Autodesk Inventor part; units mm, degrees
ref_plane "YZ Plane" through (0, 0, 0) normal (1, 0, 0) x (0, 1, 0)
ref_plane "XZ Plane" through (0, 0, 0) normal (0, 1, 0) x (-1, 0, 0)
ref_plane "XY Plane" through (0, 0, 0) normal (0, 0, 1) x (1, 0, 0)
sketch "Sketch1" plane through (0, 0, 0) normal (0, 0, 1) x (1, 0, 0)
  line L0 (-12, 5) -> (12, 5)
  line L1 (12, 5) -> (12, -5)
  line L2 (12, -5) -> (-12, -5)
  line L3 (-12, -5) -> (-12, 5)
  point P0 (0, 0)
  dimension "d0" = 24
  dimension "d1" = 10
  dimension "d2" = 5
  dimension "d3" = 12
extrude "Extrusion1" add sketch "Sketch1" along normal blind 28
sketch "Sketch2" plane through (-12, 5, 0) normal (0, 1, 0) x (1, 0, 0)
  line L0 (0, 0) -> (24, 0)
  line L1 (0, 0) -> (0, -28)
  line L2 (24, -28) -> (0, -28)
  line L3 (24, 0) -> (24, -28)
  circle A0 centre (12, -14) radius 7.5
  point P0 (12, 0)
  dimension "d6" = 15
  dimension "d7" = 28
  dimension "d8" = 24
  dimension "d9" = 12
  dimension "d10" = 14
extrude "Extrusion2" cut sketch "Sketch2" against normal up to next contours A0
sketch "Sketch7" plane through (-12, 5, 28) normal (0, 1, 0) x (1, 0, 0)
  circle A0 centre (12, 14) radius 7.5
  line L0 (0, 28) -> (0, 0)
  line L1 (24, 0) -> (0, 0)
  line L2 (24, 28) -> (24, 0)
  arc A1 (0, 14) -> (24, 14) centre (12, 14) ccw
  line L3 (24, 32) -> (24, 0)
  line L4 (24, 32) -> (24, 0)
  line L5 (24, 14) -> (24, 0)
  line L6 (24, 0) -> (0, 0)
  line L7 (24, 0) -> (0, 0)
  line L8 (0, 0) -> (0, 14)
  line L9 (0, 32) -> (0, 0)
  line L10 (0, 28) -> (24, 28)
  point P0 (12, 28)
extrude "Extrusion6" cut sketch "Sketch7" against normal blind 20 contours A1 L2 L1 L0
sketch "Sketch9" plane through (-12, -5, 0) normal (-1, 0, 0) x (0, 0, 1)
  line L0 (14, 0) -> (14, 10) construction
  line L1 (0, 10) -> (14, 10) construction
  line L2 (0, 0) -> (0, 10) construction
  line L3 (0, 0) -> (14, 0) construction
  line L4 (0, 10) -> (14, 10)
  line L5 (0, 10) -> (0, 20)
  line L6 (0, 20) -> (4, 20)
  line L7 (4, 20) -> (4, 30)
  line L8 (4, 30) -> (6, 30)
  line L9 (6, 30) -> (6, 18)
  line L10 (6, 18) -> (2, 18)
  line L11 (2, 18) -> (2, 10)
  line L12 (0, 10) -> (2, 10)
  point P0 (0, 5)
  dimension "d32" = 10
  dimension "d33" = 4
  dimension "d34" = 10
  dimension "d35" = 2
  dimension "d36" = 2
  dimension "d37" = 2
extrude "Extrusion8" add sketch "Sketch9" against normal up to surface (24 mm away)
equation "\"d9\" = 0.5 * d8"
equation "\"d10\" = 0.5 * d7"
properties part number "ProbeMount"
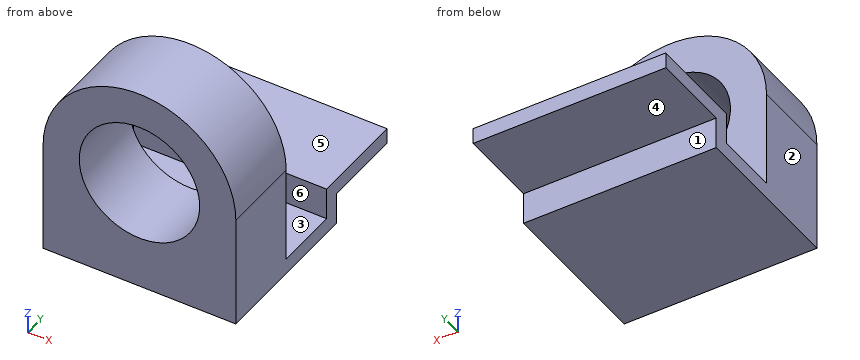
Work out the finished part from the listing and answer in its coordinate system (mm). Face numbers are marked on the shaded views. A direction names the side the tool comes from. Give positions to 0.01 mm unless a question says otherwise; leave off trailing zeros. Order: outer loops, then holes, each group sorted by start corner. A loop starts at its lowest first (then second) coordinate and runs counter-clockwise, first axis right, second up. Notation, with made-up numbers: (-18.5, 82) -> (27.5, 82) arc R24 ccw to (27.5, 118) -> close; hole circle Ø8 at (11, 87.5). An arc over 180 degrees is marked (long way). Answer as a JSON object with one key per item and string values. Group by question number.
1. A tool of negligible diameter and unlimited length cuts with its end or side. For the marked faces 4, 5 and 6, from which of +Z, -Z, +X, -X, +Y, -Y can it reach the whole face along a straight path? Write none if from no direction.
2. Flat-ended cylindrical pins translate along their axes: pin 1 Ø4 at (x, y) = (-8.5, 10.5) entering from +Z; pin 2 Ø1.2 at (x, z) = (-4, 2) entering from +Y; pin 3 Ø1.5 at (x, z) = (2, 20) entering from +Y; pin 4 Ø9.5 at (x, y) = (-3.5, 21.5) entering from +Z. Find the tip coordinate at first contact, or state that the pin passes through.
3. Section C-C on z = 19 is taken. Determine the outline of the cut face in (x, y).
4. Consider line 1 along Z through (x, y) = (0, -0.25); line 2 along X through (y, z) = (-0.5, 14); line 3 along Z through (x, y) = (8.5, 11.75). Determine where each line is inside the solid, lowest interval first. Write a range as [from, to].
5. Section D-D on x = 10.25 is taken. Determine the outline of the cut face in (y, z), plus the area to 3 significant figures.
6. The mould has two halves that part along Y. Classify the marked faces 1, 2 and 3: released by +Y, released by -Y, zero draft, split by the parting line, or undercut.
7. Section B-B on y = -0.75 is taken. Determine the outline of the cut face in (x, z).
8. Section A-A on x = 0 is taken. Determine the outline of the cut face in (y, z).
Result sheet:
{
 "1": {"face 4": "-Z, +X, -X, +Y", "face 5": "+Z, +X, -X, +Y", "face 6": "+Z, +X, -X"},
 "2": {"pin 1": "stops at z = 2", "pin 2": "stops at y = 15", "pin 3": "passes through", "pin 4": "stops at z = 6"},
 "3": {"outline": "(-10.91, -5) -> (-5.59, -5) -> (-5.59, 5) -> (-10.91, 5) -> close; (5.59, -5) -> (10.91, -5) -> (10.91, 5) -> (5.59, 5) -> close"},
 "4": {"line 1": "z = [0, 6.5], [21.5, 26]", "line 2": "x = [-12, -7.5], [7.5, 12]", "line 3": "z = [0, 2]"},
 "5": {"outline": "(-5, 0) -> (15, 0) -> (15, 4) -> (25, 4) -> (25, 6) -> (13, 6) -> (13, 2) -> (5, 2) -> (5, 20.24) -> (-5, 20.24) -> close", "area": "250 mm^2"},
 "6": {"face 1": "released by +Y", "face 2": "zero draft", "face 3": "undercut"},
 "7": {"outline": "(-12, 0) -> (12, 0) -> (12, 14) arc R12 ccw to (-12, 14) -> close; hole circle Ø15 at (0, 14)"},
 "8": {"outline": "(-5, 0) -> (15, 0) -> (15, 4) -> (25, 4) -> (25, 6) -> (13, 6) -> (13, 2) -> (5, 2) -> (5, 6.5) -> (-5, 6.5) -> close; (-5, 21.5) -> (5, 21.5) -> (5, 26) -> (-5, 26) -> close"}
}
